Verification items for this drawing (mm, ordinates from the low corner). Coordinates: 2 decimals unless noted, no trailing zeros. Write each loop counter-clockwise with the first axis right and the second up, starting at its lowest first coordinate (ties: lowest second). Pieces come first, ordered by that corner, then holes.
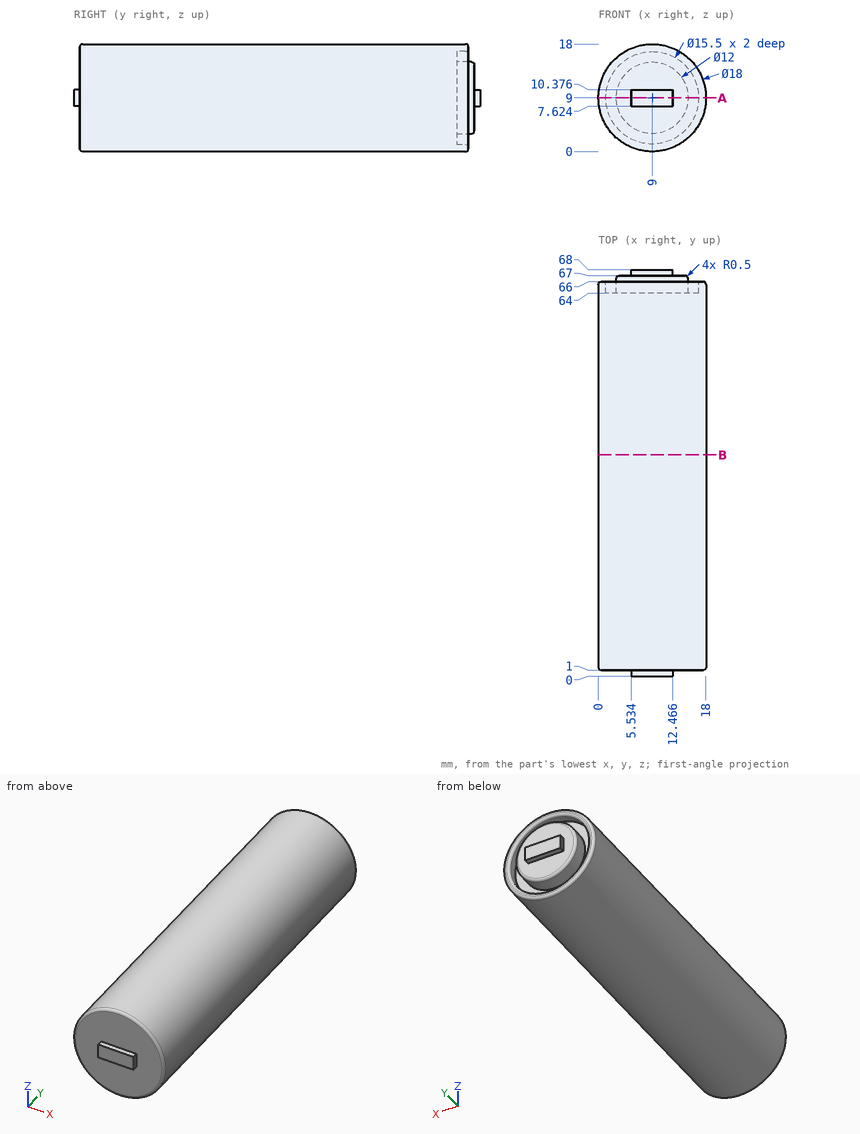
1. Gauge pin test, flat ends, axial feed: pin 1 Ø5.5 at (x, z) = (8.5, 7) entering from +Y; pin 2 Ø0.5 at (x, y) = (8, 0.5) entering from -Z; pin 3 Ø0.5 at (y, z) = (0.5, 9.5) entering from +X; pin 4 Ø6 at (y, z) = (45, 4.5) entering from +X. Record the tip position at first contact, or that the pin passes through.
Computed values:
pin 1: stops at y = 68
pin 2: stops at z = 7.62
pin 3: stops at x = 12.47
pin 4: stops at x = 17.87
2. Sectioned sample at B-B, the plane y = 37. Record the boundary of the cut face in (x, z).
Computed values:
outline: circle Ø18 at (9, 9)
3. Sectioned sample at A-A, the plane z = 9. Record the boundary of the cut face in (x, y).
Computed values:
outline: (0, 1.5) arc R0.5 ccw to (0.5, 1) - (5.53, 1) - (5.53, 0) - (12.47, 0) - (12.47, 1) - (17.5, 1) arc R0.5 ccw to (18, 1.5) - (18, 65.5) arc R0.5 ccw to (17.5, 66) - (17.25, 66) arc R0.5 ccw to (16.75, 65.5) - (16.75, 64) - (15, 64) - (15, 66.5) arc R0.5 ccw to (14.5, 67) - (12.47, 67) - (12.47, 68) - (5.53, 68) - (5.53, 67) - (3.5, 67) arc R0.5 ccw to (3, 66.5) - (3, 64) - (1.25, 64) - (1.25, 65.5) arc R0.5 ccw to (0.75, 66) - (0.5, 66) arc R0.5 ccw to (0, 65.5) - close
4. Thickness scan on line 1 along X through (y, z) = (65, 9); line 2 along Z through (x, y) = (4.5, 65.5) (1 decimal); line 3 along Y through (x, z) = (9.75, 13.5). Record the ranges inside material, lowest first.
Computed values:
line 1: x = 0 to 1.25, 3 to 15, 16.75 to 18
line 2: z = 1.2 to 2.7, 5 to 13, 15.3 to 16.8
line 3: y = 1 to 67
